```python
from build123d import *

# Parameters (mm, degrees)
F1_DEPTH = 38.1


with BuildPart() as f1:
    # F0 (on Top) → F1 (new body, symmetric)
    with BuildSketch(Plane.XY):
        Polygon((7.81685, 0), (-1.32715, 0), (0, -4.63993), (-2.54, -4.63993), (-2.54, -80.83993), (-27.94, -80.83993), (-27.94, -85.91993), (34.4297, -85.91993), (34.4297, -80.83993), (9.0297, -80.83993), (9.0297, -4.63993), (6.4897, -4.63993), align=None)
    extrude(amount=F1_DEPTH, both=True)


with BuildPart() as f1_1:
    # F2: moved
    add(f1.part.moved(Location((-4.064, 44.958, 0))))


solid = f1_1.part
```
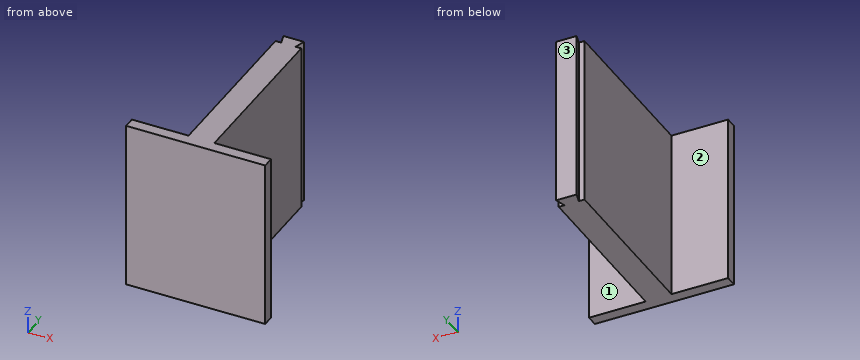
Read the model definition and answer for the solid it produces. Units are mm, in the model's axes. Face numbers are marked on the shaded views. A direction names the side the tool comes from. Give positions to 0.01 mm unless a question says otherwise; leave off trailing zeros. Loops run counter-clockwise (first coordinate to the right, second up) from the corner with the lowest first, then second, coordinate; pieces in that order, holes last.
Item 1: The part is cut by section B-B (x = -25). Write down the section's boundary in (y, z).
Item 2: Find the intervals of material crossed by line 1 along Y through (x, z) = (-25, -18); line 2 along X through (y, z) = (-27.5, -34.5), in increasing order.
Item 3: The part is cut by section C-C (y = 31.5). Write down the section's boundary in (x, z).
Item 4: The part is cut by section A-A (z = -14.5). Write down the section's boundary in (x, y), and give its area (3 significant figures).
Item 5: For the marked faces 1, 2 and 3, determine the directions among +Z, -Z, +X, -X, +Y, -Y from which every point of the face is accessible in a straight line to the end or side of a thin tool.
Item 6: Each of these flat-tipped pins is pushed along its axis until it touches: pin 1 Ø3 at (x, z) = (23, -27) entering from +Y; pin 2 Ø2 at (x, z) = (-6, -3.5) entering from +Y; pin 3 Ø5 at (y, z) = (-6.5, -17) entering from +X; pin 4 Ø4 at (y, z) = (-23.5, 22.5) entering from -X. Where does it stop, or does it pass through?
Taken from the geometry:
1. outline: (-40.96, -38.1) - (-35.88, -38.1) - (-35.88, 38.1) - (-40.96, 38.1) - close
2. line 1: y = -40.96 to -35.88
2. line 2: x = -6.6 to 4.97
3. outline: (-6.6, -38.1) - (4.97, -38.1) - (4.97, 38.1) - (-6.6, 38.1) - close
4. outline: (-32, -40.96) - (30.37, -40.96) - (30.37, -35.88) - (4.97, -35.88) - (4.97, 40.32) - (2.43, 40.32) - (3.75, 44.96) - (-5.39, 44.96) - (-4.06, 40.32) - (-6.6, 40.32) - (-6.6, -35.88) - (-32, -35.88) - close
4. area: 1,230 mm2
5. face 1: +Z, -Z, +X, +Y
5. face 2: +Z, -Z, -X, +Y
5. face 3: +Z, -Z, +X, -X, +Y
6. pin 1: stops at y = -35.88
6. pin 2: stops at y = 44.96
6. pin 3: stops at x = 4.97
6. pin 4: stops at x = -6.6
